The listing builds one solid part. Answer for the finished solid, in the listing's coordinates (mm). Face numbers are marked on the shaded views. A direction names the side the tool comes from. Round coordinates to 2 decimals unless told otherwise and drop trailing zeros. Loops run counter-clockwise (first coordinate to the right, second up) from the corner with the lowest first, then second, coordinate; pieces in that order, holes last. Notation, with made-up numbers: (-19, 36) -> (35, 36) arc R11 ccw to (35, 49) -> close; hole circle Ø6 at (-28.5, 40). An arc over 180 degrees is marked (long way). Answer in a Markdown table with one row per item. Add a question column.
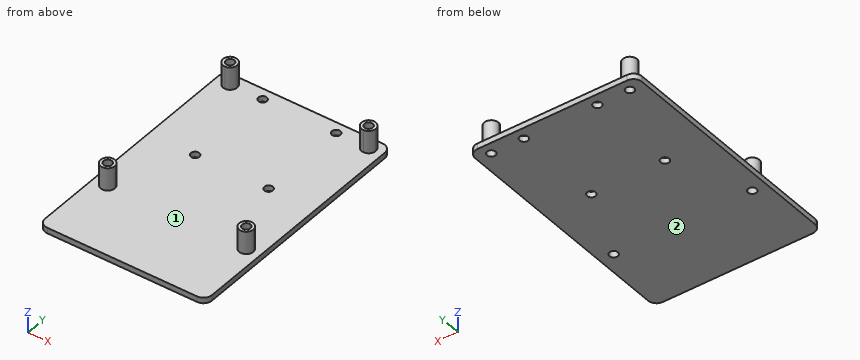
```python
from build123d import *

# Parameters (mm, degrees)
SKETCH1_W           = 59
SKETCH1_H           = 88
SKETCH1_R           = 1.5
SKETCH1_R_2         = 2.5
BOSS_EXTRUDE1_DEPTH = 2
BOSS_EXTRUDE2_DEPTH = 10
FILLET1_R           = 3


with BuildPart() as part:
    # Sketch1 → Boss-Extrude1 (new body)
    with BuildSketch(Plane.XY):
        with Locations((0, -24)):
            Rectangle(SKETCH1_W, SKETCH1_H)
        with Locations((-13, 16)):
            Circle(SKETCH1_R, mode=Mode.SUBTRACT)
        with Locations((13, 16)):
            Circle(SKETCH1_R, mode=Mode.SUBTRACT)
        with Locations((13, -16)):
            Circle(SKETCH1_R, mode=Mode.SUBTRACT)
        with Locations((-13, -16)):
            Circle(SKETCH1_R, mode=Mode.SUBTRACT)
        with Locations((-24.5, 16)):
            Circle(SKETCH1_R_2, mode=Mode.SUBTRACT)
        with Locations((24.5, 16)):
            Circle(SKETCH1_R_2, mode=Mode.SUBTRACT)
        with Locations((24.5, -42)):
            Circle(SKETCH1_R_2, mode=Mode.SUBTRACT)
        with Locations((-24.5, -42)):
            Circle(SKETCH1_R_2, mode=Mode.SUBTRACT)
    extrude(amount=BOSS_EXTRUDE1_DEPTH)

    # Sketch1_3 → Boss-Extrude2 (add)
    with BuildSketch(Plane.XY):
        with BuildLine():
            ThreePointArc((-24.5, 13.5), (-22.732233047, 14.232233047), (-22, 16))
            Line((-22, 16), (-23, 16))
            ThreePointArc((-23, 16), (-23.439339828, 14.939339828), (-24.5, 14.5))
            Line((-24.5, 14.5), (-24.5, 13.5))
        make_face()
        with BuildLine():
            Line((-23, 16), (-22, 16))
            ThreePointArc((-22, 16), (-26.267766953, 17.767766953), (-24.5, 13.5))
            Line((-24.5, 13.5), (-24.5, 14.5))
            ThreePointArc((-24.5, 14.5), (-25.560660172, 17.060660172), (-23, 16))
        make_face()
        with BuildLine():
            ThreePointArc((27, 16), (24.5, 18.5), (22, 16))
            Line((22, 16), (23, 16))
            ThreePointArc((23, 16), (24.5, 17.5), (26, 16))
            ThreePointArc((26, 16), (25.560660172, 14.939339828), (24.5, 14.5))
            Line((24.5, 14.5), (24.5, 13.5))
            ThreePointArc((24.5, 13.5), (26.267766953, 14.232233047), (27, 16))
        make_face()
        with BuildLine():
            Line((23, 16), (22, 16))
            ThreePointArc((22, 16), (22.732233047, 14.232233047), (24.5, 13.5))
            Line((24.5, 13.5), (24.5, 14.5))
            ThreePointArc((24.5, 14.5), (23.439339828, 14.939339828), (23, 16))
        make_face()
        with BuildLine():
            ThreePointArc((-22, -42), (-22.732233047, -40.232233047), (-24.5, -39.5))
            Line((-24.5, -39.5), (-24.5, -40.5))
            ThreePointArc((-24.5, -40.5), (-23.439339828, -40.939339828), (-23, -42))
            Line((-23, -42), (-22, -42))
        make_face()
        with BuildLine():
            Line((-24.5, -40.5), (-24.5, -39.5))
            ThreePointArc((-24.5, -39.5), (-26.267766953, -43.767766953), (-22, -42))
            Line((-22, -42), (-23, -42))
            ThreePointArc((-23, -42), (-25.560660172, -43.060660172), (-24.5, -40.5))
        make_face()
        with BuildLine():
            ThreePointArc((27, -42), (26.267766953, -40.232233047), (24.5, -39.5))
            Line((24.5, -39.5), (24.5, -40.5))
            ThreePointArc((24.5, -40.5), (25.560660172, -40.939339828), (26, -42))
            ThreePointArc((26, -42), (24.5, -43.5), (23, -42))
            Line((23, -42), (22, -42))
            ThreePointArc((22, -42), (24.5, -44.5), (27, -42))
        make_face()
        with BuildLine():
            Line((24.5, -40.5), (24.5, -39.5))
            ThreePointArc((24.5, -39.5), (22.732233047, -40.232233047), (22, -42))
            Line((22, -42), (23, -42))
            ThreePointArc((23, -42), (23.439339828, -40.939339828), (24.5, -40.5))
        make_face()
    extrude(amount=BOSS_EXTRUDE2_DEPTH)

    # Fillet1
    fillet1_edges = [part.edges().sort_by_distance(p)[0] for p in [
        (29.5, -68, 1),
        (-29.5, -68, 1),
        (-29.5, 20, 1),
        (29.5, 20, 1),
    ]]
    fillet(fillet1_edges, radius=FILLET1_R)


solid = part.part
```
Item 1: Flat-ended cylindrical pins translate along their axes: P1, Ø1, axis at x = 12, y = -7, coming from the +Z side; P2, Ø2.5, axis at x = -24.5, y = 16, coming from the -Z side; P3, Ø4, axis at x = 23, z = 7, coming from the +Y side; P4, Ø8, axis at x = 11.5, y = -46, coming from the -Z side. Find the tip coordinate at first contact, or state that the pin passes through.
Item 2: Section C-C, the plane y = -16 is taken. Write down the section's boundary in (x, z), and give its area (3 significant figures).
Item 3: Consider L1, parallel to X at y = 16, z = 2.25; L2, parallel to Y at x = -24.5, z = 6; L3, parallel to Y at x = 13, z = 1. Determine where each line is inside the solid, lowest interval first. Write a range as from..to.
Item 4: Section A-A, the plane x = 13 is taken. Write down the section's boundary in (y, z).
Item 5: Section B-B, the plane z = 5.75 is taken. Write down the section's boundary in (x, y).
Item 6: For the marked faces 1 and 2, determine the directions among +Z, -Z, +X, -X, +Y, -Y from which every point of the face is accessible in a straight line to the end or side of a thin tool.
Item 7: Section D-D, the plane x = 20 is taken. Write down the section's boundary in (y, z), and give its area (3 significant figures).
Here are the results:
| question | item | result |
|---|---|---|
| 1 | P1 | stops at z = 2 |
| 1 | P2 | passes through |
| 1 | P3 | stops at y = 18.5 |
| 1 | P4 | stops at z = 0 |
| 2 | outline | (-29.5, 0) -> (-14.5, 0) -> (-14.5, 2) -> (-29.5, 2) -> close; (-11.5, 0) -> (11.5, 0) -> (11.5, 2) -> (-11.5, 2) -> close; (14.5, 0) -> (29.5, 0) -> (29.5, 2) -> (14.5, 2) -> close |
| 2 | area | 106 mm² |
| 3 | L1 | x = -27..-26, -23..-22, 22..23, 26..27 |
| 3 | L2 | y = -44.5..-43.5, -40.5..-39.5, 13.5..14.5, 17.5..18.5 |
| 3 | L3 | y = -68..-17.5, -14.5..14.5, 17.5..20 |
| 4 | outline | (-68, 0) -> (-17.5, 0) -> (-17.5, 2) -> (-68, 2) -> close; (-14.5, 0) -> (14.5, 0) -> (14.5, 2) -> (-14.5, 2) -> close; (17.5, 0) -> (20, 0) -> (20, 2) -> (17.5, 2) -> close |
| 5 | outline | circle Ø5 at (-24.5, -42); circle Ø5 at (-24.5, 16); circle Ø5 at (24.5, -42); circle Ø5 at (24.5, 16); hole circle Ø3 at (-24.5, -42); hole circle Ø3 at (-24.5, 16); hole circle Ø3 at (24.5, -42); hole circle Ø3 at (24.5, 16) |
| 6 | face 1 | +Z |
| 6 | face 2 | -Z, +X, -X, +Y, -Y |
| 7 | outline | (-68, 0) -> (20, 0) -> (20, 2) -> (-68, 2) -> close |
| 7 | area | 176 mm² |
